For this review, use the dimensioned drawing (mm, ordinates from the lowest corner) and the shaded views. A direction names the side the tool comes from. Coordinates: 2 decimals unless noted, no trailing zeros. Order: outer loops, then holes, each group sorted by start corner. A loop starts at its lowest first (then second) coordinate and runs counter-clockwise, first axis right, second up. Notation, with made-up numbers: (13, 84) -> (40, 84) arc R20 cw to (40, 95) -> close; hole circle Ø10 at (77.25, 64). An arc over 180 degrees is marked (long way). Use one line per item in the form item = value. Start each with the question number.
(1) Take a section at B-B (x = 82.55). State the section outline as (y, z) points.
(2) Take a section at A-A (z = 72.39). State the section outline as (x, y) points, then the cut area to 3 significant figures.
(3) Insertion check: pin 1 Ø5 at (x, z) = (59.5, 37.5) entering from +Y; pin 2 Ø3 at (y, z) = (19, 35.5) entering from -X; pin 3 Ø2 at (y, z) = (21, 35) entering from +X. Each pin has a flat end and moves straight along its axis. Give the tip position at first contact, or say it passes through.
(4) For the marked faces 1 and 2, list the 3-axis set-ups (+Z, -Z, +X, -X, +Y, -Y) from which the entire face can be reached by the end or side of a thin tool; tool diameter is ignored.
(5) Wall thickness on line 1 along Z through (x, y) = (3.81, 1.1); line 2 along X through (y, z) = (0.9, 72.39); line 3 along Z through (x, y) = (82, 1): over which ranges is each line inside the solid? List them lowest first.
(6) Take a section at C-C (x = 26). State the section outline as (y, z) points, then the cut area to 3 significant figures.
(7) Take a section at D-D (y = 5.5). State the section outline as (x, z) points.
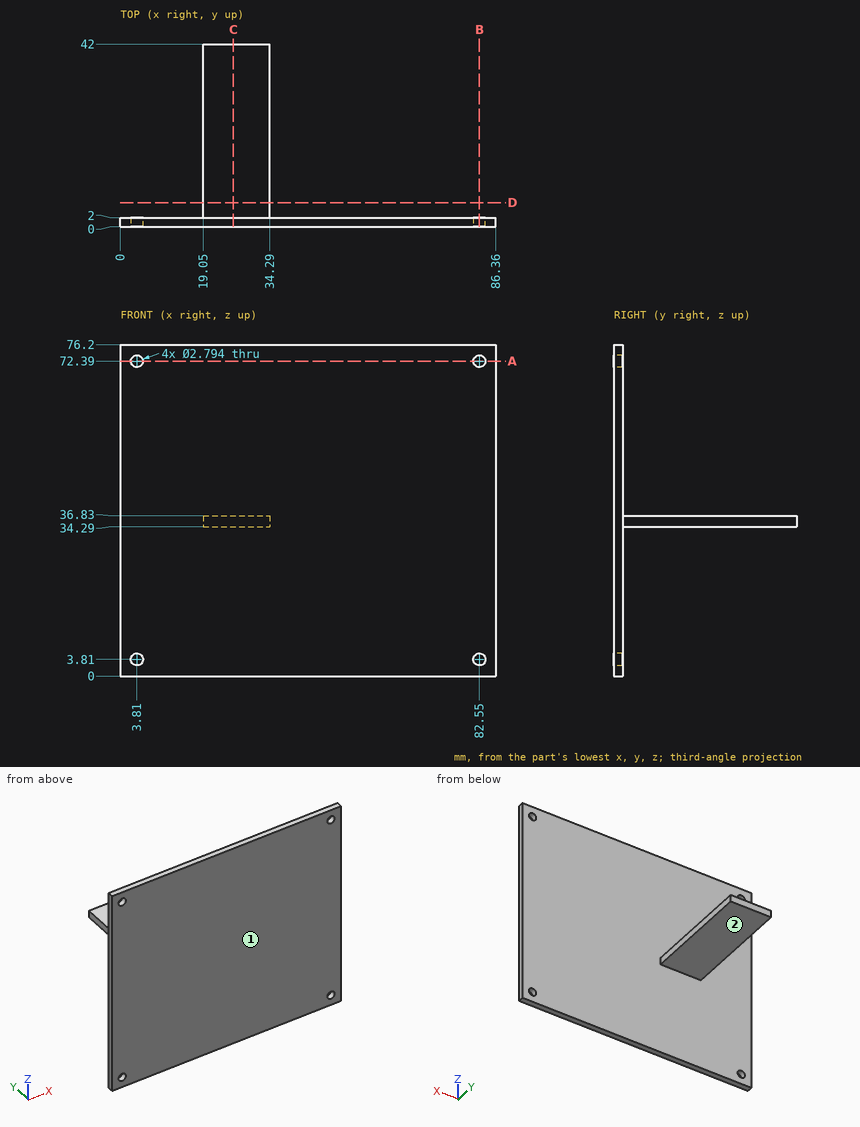
Findings:
q1.outline = (0, 0) -> (2, 0) -> (2, 2.41) -> (0, 2.41) -> close; (0, 5.21) -> (2, 5.21) -> (2, 70.99) -> (0, 70.99) -> close; (0, 73.79) -> (2, 73.79) -> (2, 76.2) -> (0, 76.2) -> close
q2.outline = (0, 0) -> (2.41, 0) -> (2.41, 2) -> (0, 2) -> close; (5.21, 0) -> (81.15, 0) -> (81.15, 2) -> (5.21, 2) -> close; (83.95, 0) -> (86.36, 0) -> (86.36, 2) -> (83.95, 2) -> close
q2.area = 162 mm²
q3.pin_1 = 2
q3.pin_2 = 19.05
q3.pin_3 = 34.29
q4.face_1 = +Z, -Z, +X, -X, -Y
q4.face_2 = -Z, +X, -X, +Y
q5.line_1 = 0 to 2.41, 5.21 to 70.99, 73.79 to 76.2
q5.line_2 = 0 to 2.41, 5.21 to 81.15, 83.95 to 86.36
q5.line_3 = 0 to 2.53, 5.09 to 71.11, 73.67 to 76.2
q6.outline = (0, 0) -> (2, 0) -> (2, 34.29) -> (42, 34.29) -> (42, 36.83) -> (2, 36.83) -> (2, 76.2) -> (0, 76.2) -> close
q6.area = 254 mm²
q7.outline = (19.05, 34.29) -> (34.29, 34.29) -> (34.29, 36.83) -> (19.05, 36.83) -> close
